For this review, use the dimensioned drawing (mm, ordinates from the lowest corner) and the shaded views. A direction names the side the tool comes from. Coordinates: 2 decimals unless noted, no trailing zeros. Order: outer loops, then holes, each group sorted by start corner. A loop starts at its lowest first (then second) coordinate and runs counter-clockwise, first axis right, second up. Notation, with made-up numbers: M 9.25,5 L 65.25,5 A12 ccw 65.25,24 Z; hole C 6,-19.75 d3. An arc over 180 degrees is marked long. Answer in a Markdown table with one row per item.
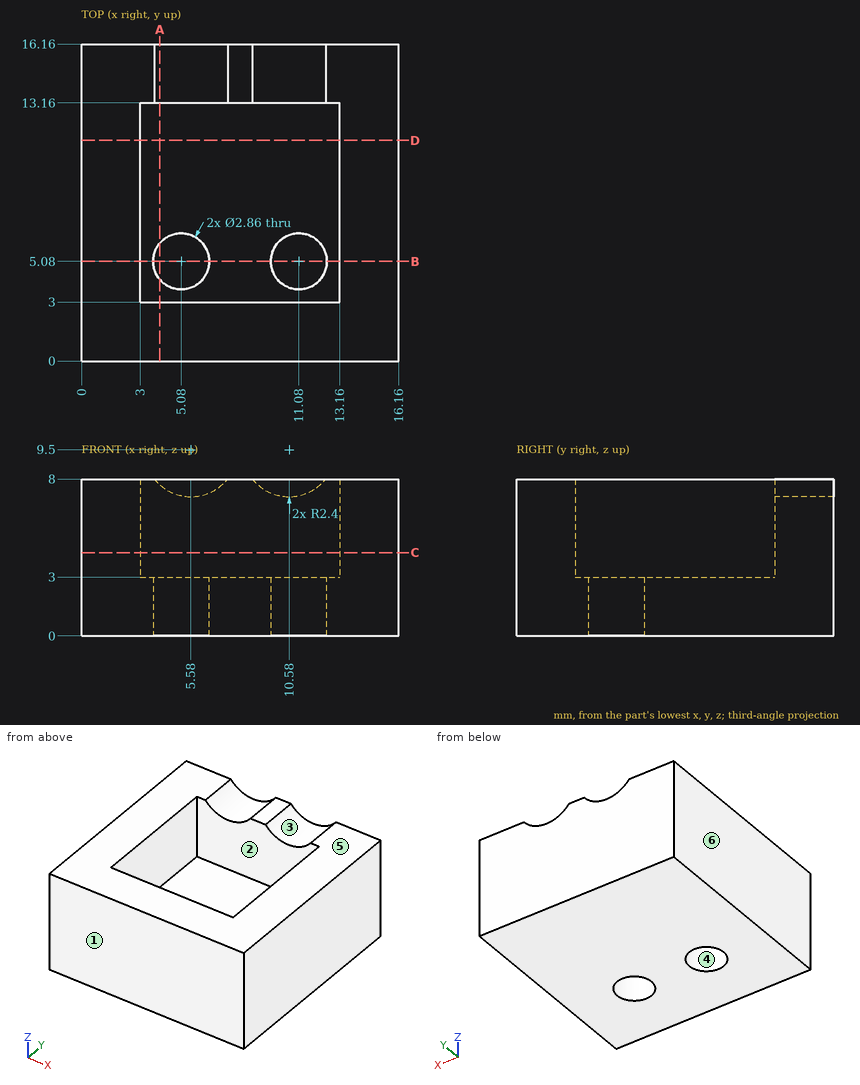
(1) Take a section at D-D (y = 11.25). Write out the cut boundary in (x, z), then the cut area to 3 significant figures.
Report:
| item | result |
|---|---|
| outline | M 0,0 L 16.16,0 L 16.16,8 L 13.16,8 L 13.16,3 L 3,3 L 3,8 L 0,8 Z |
| area | 78.5 mm^2 |
(2) Take a section at B-B (y = 5.08). Write out the cut boundary in (x, z).
Report:
| item | result |
|---|---|
| outline | M 0,0 L 3.65,0 L 3.65,3 L 3,3 L 3,8 L 0,8 Z; M 6.51,0 L 9.65,0 L 9.65,3 L 6.51,3 Z; M 12.51,0 L 16.16,0 L 16.16,8 L 13.16,8 L 13.16,3 L 12.51,3 Z |
(3) The part is to be moulded in two halves that separate along X. For the marked faces 4, 5 and 6, say which applies: +X half, -X half, draft (parallel to the pull), parting line (faces both ways), or undercut.
Report:
| item | result |
|---|---|
| face 4 | undercut |
| face 5 | draft |
| face 6 | -X half |
(4) Take a section at A-A (x = 4). Write out the cut boundary in (y, z), then the cut area to 3 significant figures.
Report:
| item | result |
|---|---|
| outline | M 0,0 L 4.14,0 L 4.14,3 L 3,3 L 3,8 L 0,8 Z; M 6.02,0 L 16.16,0 L 16.16,7.69 L 13.16,7.69 L 13.16,3 L 6.02,3 Z |
| area | 71.9 mm^2 |
(5) Insertion check: P1, Ø3.5, axis at x = 11.08, y = 5.08, coming from the +Z side. The pin has a flat end and moves straight along its axis. Give the tip position at first contact, or say it passes through.
Report:
| item | result |
|---|---|
| P1 | z = 3 |
(6) Machinability: for the marked faces 1, 2 and 3, which of the approach directions +Z, -Z, +X, -X, +Y, -Y give a long, thin tool a straight path to every point of the face, cutting with its end or side? Answer none if there is none.
Report:
| item | result |
|---|---|
| face 1 | +Z, -Z, +X, -X, -Y |
| face 2 | +Z |
| face 3 | +Z, +Y |
(7) To check wall thickness, follow line 1 (X direction, y = 5.08, z = 1.3); line 2 (Y direction, x = 6.5, z = 5.5). State the ranges of each line that lie inside material, in increasing order. Write a range as [from, to].
Report:
| item | result |
|---|---|
| line 1 | [0, 3.65], [6.51, 9.65], [12.51, 16.16] |
| line 2 | [0, 3], [13.16, 16.16] |
(8) Take a section at C-C (z = 4.25). Write out the cut boundary in (x, y), then the cut area to 3 significant figures.
Report:
| item | result |
|---|---|
| outline | M 0,0 L 16.16,0 L 16.16,16.16 L 0,16.16 Z; hole M 3,3 L 13.16,3 L 13.16,13.16 L 3,13.16 Z |
| area | 158 mm^2 |
